Check sheet for the drawn part. Datum: minimum x, y, z corner. Units: mm. Round coordinates to 2 decimals unless told otherwise and drop trailing zeros. Write each loop counter-clockwise with the first axis right and the second up, starting at its lowest first coordinate (ties: lowest second). Pieces come first, ordered by that corner, then holes. Notation, with made-up numbers: (-29.5, -16) - (1.5, -16) arc R16 cw to (1.5, 15) - close; hole circle Ø3 at (37.5, -10.75). An arc over 180 degrees is marked (long way). Answer as a JSON object with one key per item and string values.
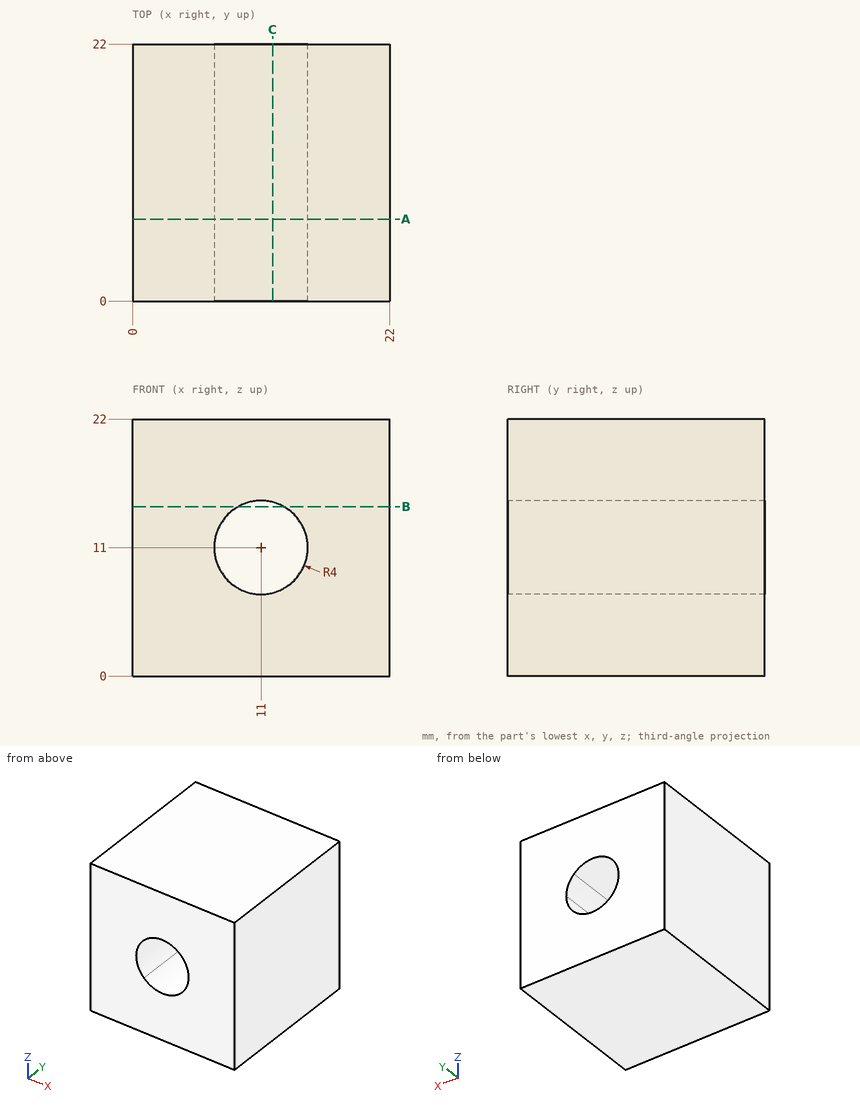
1. Cross-section at B-B (z = 14.5). Record the boundary of the cut face in (x, y).
Completed:
{"outline": "(0, 0) - (9.06, 0) - (9.06, 22) - (0, 22) - close; (12.94, 0) - (22, 0) - (22, 22) - (12.94, 22) - close"}
2. Cross-section at C-C (x = 12). Record the boundary of the cut face in (y, z), plus the area to 3 significant figures.
Completed:
{"outline": "(0, 0) - (22, 0) - (22, 7.13) - (0, 7.13) - close; (0, 14.87) - (22, 14.87) - (22, 22) - (0, 22) - close", "area": "314 mm^2"}
3. Cross-section at A-A (y = 7). Record the boundary of the cut face in (x, z).
Completed:
{"outline": "(0, 0) - (22, 0) - (22, 22) - (0, 22) - close; hole circle Ø8 at (11, 11)"}
4. Material ranges on probe 1 along Z at (x, y) = (11, 1); probe 2 along X at (y, z) = (2.5, 12.25); probe 3 along X at (y, z) = (1, 13.25), recorded low to high. Write a range as from..to.
Completed:
{"probe 1": "z = 0..7, 15..22", "probe 2": "x = 0..7.2, 14.8..22", "probe 3": "x = 0..7.69, 14.31..22"}
